Read the model definition and answer for the solid it produces. Units are mm, in the model's axes. Give positions to 0.01 mm unless a question says otherwise; leave off trailing zeros. Write each loop counter-clockwise with the first axis right and the second up, starting at its lowest first coordinate (ties: lowest second). Pieces come first, ordered by that corner, then holes. Notation, with made-up numbers: (15, 62.25) - (50, 62.25) arc R28 cw to (50, 83.25) - close; hole circle Ø8 at (47.5, 21). An arc over 180 degrees is marked (long way). Answer as a JSON object with one key per item and string values. Group by question number.
Solid Edge part; units mm, degrees
sketch "Sketch1" plane through (0, 0, 0) normal (0, -1, 0) x (1, 0, 0)
  arc A0 (0, 0) -> (940, 940) centre (940, 0) cw
  line L0 (940, 940) -> (1698, 940)
  line L1 (1698, 940) -> (1698, 0)
sketch "Sketch2" plane through (0, 0, 0) normal (0, 0, 1) x (1, 0, 0)
  line L0 (-20, -10) -> (20, -10)
  line L1 (20, -10) -> (20, 10)
  line L2 (20, 10) -> (-20, 10)
  line L3 (-20, 10) -> (-20, -10)
sweep "ÁtvezetettKihúzás_1" add profiles "Sketch2" path "Sketch1"
extrude "Kihúzás_1" [suppressed]
extrude "Kihúzás_2" [suppressed]
fillet "Lekerekítés_1" [suppressed]
revolve "RevolvedProtrusion1" [suppressed]
1) Find section B-B, the plane y = 6.25. Write down the section's boundary in (x, z).
2) Flat-ended cylindrical pins translate along their axes: pin 1 Ø8 at (x, y) = (187, 6.5) entering from -Z; pin 2 Ø10 at (x, y) = (1179, 5) entering from -Z; pin 3 Ø10 at (x, y) = (769, 3) entering from -Z. Find the tip coordinate at first contact, or state that the pin passes through.
3) Find the intervals of material crossed by line 1 (Z direction, x = 1117, y = 0); line 2 (X direction, y = 6.25, z = 98); line 3 (X direction, y = -7.5, z = 251), in increasing order. Write a range as [from, to].
4) For a pull along X with two mould halves and no side action, classify faces 1 (the cylindrical face through (268.682, -0.14, 686.245)), 2 (the flat face through (972, -10, 950)), 3 (the cylindrical face through (282.35, 0.14, 643.35)) as released by +X, released by -X, zero draft, split by the parting line, or undercut.
5) Find section C-C, the plane z = 398. Write down the section's boundary in (x, y).
6) Find section D-D, the plane x = 981.5. Write down the section's boundary in (y, z).
7) Find section A-A, the plane z = 589. Write down the section's boundary in (x, y).
Values follow:
{
 "1": {"outline": "(-20, 0) - (20, 0) arc R920 cw to (940, 920) - (1678, 920) - (1678, 0) - (1718, 0) - (1718, 960) - (940, 960) arc R960 ccw to start"},
 "2": {"pin 1": "stops at z = 522.83", "pin 2": "stops at z = 920", "pin 3": "stops at z = 903.01"},
 "3": {"line 1": "z = [920, 960]", "line 2": "x = [-14.98, 25.23], [1678, 1718]", "line 3": "x = [13.39, 54.9], [1678, 1718]"},
 "4": {"face 1": "released by -X", "face 2": "zero draft", "face 3": "undercut"},
 "5": {"outline": "(66.39, -10) - (110.54, -10) - (110.54, 10) - (66.39, 10) - close; (1678, -10) - (1718, -10) - (1718, 10) - (1678, 10) - close"},
 "6": {"outline": "(-10, 920) - (10, 920) - (10, 960) - (-10, 960) - close"},
 "7": {"outline": "(181.92, -10) - (233.26, -10) - (233.26, 10) - (181.92, 10) - close; (1678, -10) - (1718, -10) - (1718, 10) - (1678, 10) - close"}
}
